Verification items for this drawing (mm, ordinates from the low corner). A direction names the side the tool comes from. Give positions to 0.01 mm unless a question says otherwise; leave off trailing zeros. Order: outer loops, then holes, each group sorted by start corner. A loop starts at its lowest first (then second) coordinate and runs counter-clockwise, first axis right, second up.
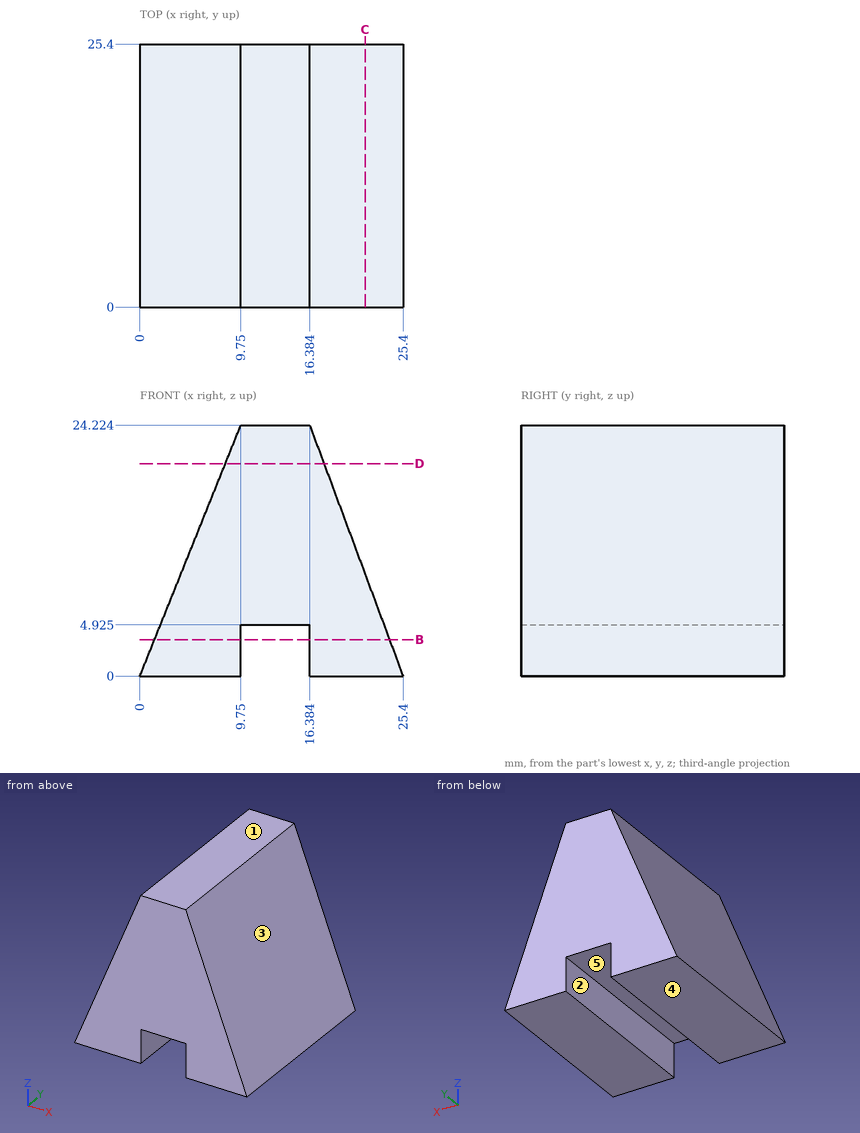
Q1. Release check for a two-part mould opening along X. For the marked faces 1, 2 and 3 record: pulls with the +X half, pulls with the -X half, needs draft (parallel to the pull), parting line crosses it, or undercut.
Q2. Gauge pin test, flat ends, axial feed: P1, Ø6, axis at y = 19, z = 11.5, coming from the +X side; P2, Ø6, axis at y = 11, z = 5.5, coming from the -X side; P3, Ø4, axis at y = 11.5, z = 3.5, coming from the +X side. Record the tip position at first contact, or that the pin passes through.
Q3. Cross-section at B-B, the plane z = 3.5. Record the boundary of the cut face in (x, y).
Q4. Access from +Z, -Z, +X, -X, +Y, -Y to the whole of each face (thin tool, end or side, straight path). Record for the marked faces 4 and 5.
Q5. Cross-section at C-C, the plane x = 21.75. Record the boundary of the cut face in (y, z), and give its area (3 significant figures).
Q6. Thickness scan on L1, parallel to Z at x = 12.5, y = 16 (1 decimal); L2, parallel to X at y = 16.5, z = 17.25; L3, parallel to X at y = 14, z = 4.75. Record the ranges inside material, lowest first.
Q7. Cross-section at D-D, the plane z = 20.5. Record the boundary of the cut face in (x, y).
Answers follow:
1. face 1: needs draft
1. face 2: undercut
1. face 3: pulls with the +X half
2. P1: stops at x = 22.24
2. P2: stops at x = 1.01
2. P3: stops at x = 24.84
3. outline: (1.41, 0) - (9.75, 0) - (9.75, 25.4) - (1.41, 25.4) - close; (16.38, 0) - (24.1, 0) - (24.1, 25.4) - (16.38, 25.4) - close
4. face 4: -Z, +X, -X, +Y, -Y
4. face 5: -Z, +Y, -Y
5. outline: (0, 0) - (25.4, 0) - (25.4, 9.81) - (0, 9.81) - close
5. area: 249 mm2
6. L1: z = 4.9 to 24.2
6. L2: x = 6.94 to 18.98
6. L3: x = 1.91 to 9.75, 16.38 to 23.63
7. outline: (8.25, 0) - (17.77, 0) - (17.77, 25.4) - (8.25, 25.4) - close
